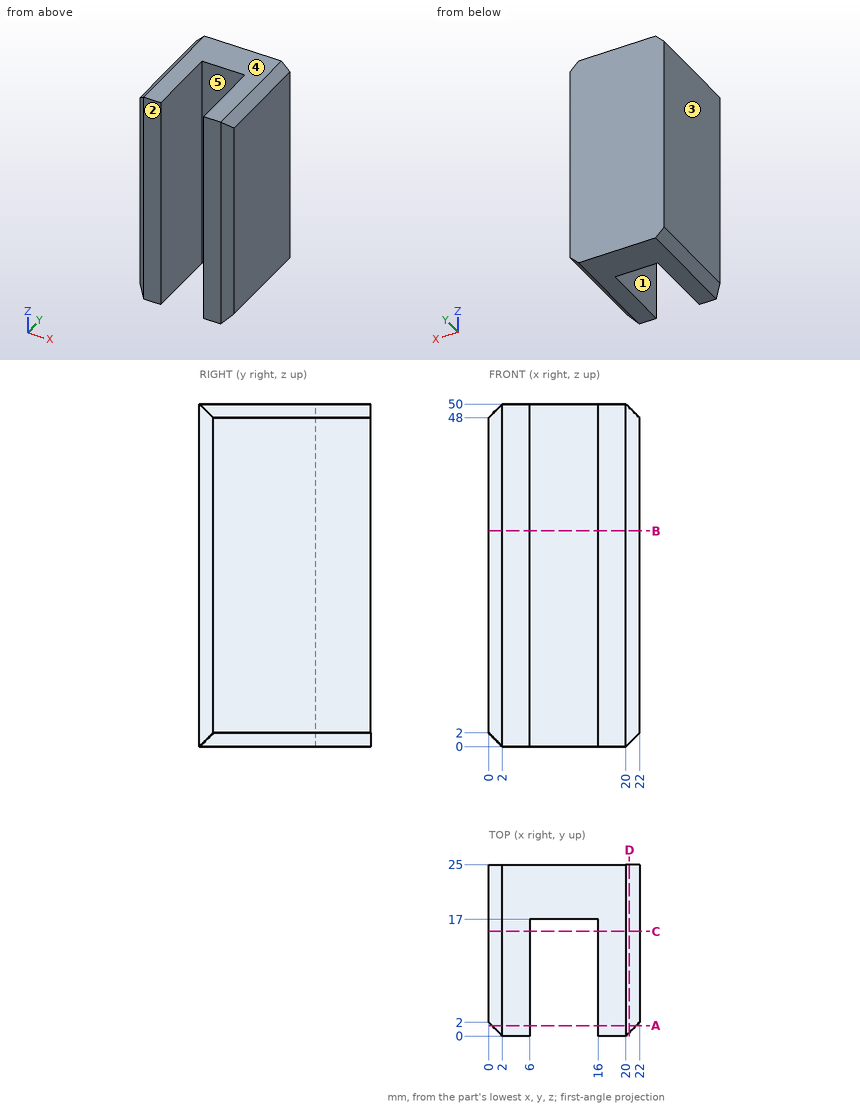
Can you work these out from the drawing? Everything is in mm from the part's minimum corner. A direction names the side the tool comes from. Round coordinates to 2 decimals unless told otherwise and drop trailing zeros. Loops run counter-clockwise (first coordinate to the right, second up) from the corner with the lowest first, then second, coordinate; pieces in that order, holes last.
1. If we section it at B-B on z = 31.5: Write out the boundary of the cut face in (x, y), plus the area to 3 significant figures.
Answer list:
outline: (0, 2) - (2, 0) - (6, 0) - (6, 17) - (16, 17) - (16, 0) - (20, 0) - (22, 2) - (22, 25) - (0, 25) - close
area: 376 mm2
2. If we section it at A-A on y = 1.5: Write out the boundary of the cut face in (x, z).
Answer list:
outline: (0.5, 1.5) - (2, 0) - (6, 0) - (6, 50) - (2, 50) - (0.5, 48.5) - close; (16, 0) - (20, 0) - (21.5, 1.5) - (21.5, 48.5) - (20, 50) - (16, 50) - close
3. We'd pull the mould along X, two halves only. Please class the marked faces 3, 4 and 5: +X half, -X half, draft (parallel to the pull), parting line (faces both ways), or undercut.
Answer list:
face 3: -X half
face 4: draft
face 5: undercut
4. If I drill on line 1 along X through (y, z) = (13.25, 12.5); line 2 along Y through (x, z) = (15.5, 12); line 3 along X through (y, z) = (1.75, 4), over which ranges is the centre line in solid material (lowest first)?
Answer list:
line 1: x = 0 to 6, 16 to 22
line 2: y = 17 to 25
line 3: x = 0.25 to 6, 16 to 21.75
5. For P1, Ø3, axis at x = 10.5, z = 16.5, coming from the -Y side, with a flat end and sliding along its axis, tell me the tip position at first contact or that it passes through.
Answer list:
P1: stops at y = 17
6. If we section it at D-D on x = 20.5: Write out the boundary of the cut face in (y, z).
Answer list:
outline: (0.5, 0.5) - (25, 0.5) - (25, 49.5) - (0.5, 49.5) - close
7. If we section it at C-C on y = 15.25: Write out the boundary of the cut face in (x, z).
Answer list:
outline: (0, 2) - (2, 0) - (6, 0) - (6, 50) - (2, 50) - (0, 48) - close; (16, 0) - (20, 0) - (22, 2) - (22, 48) - (20, 50) - (16, 50) - close
8. Which directions (+Z, -Z, +X, -X, +Y, -Y) give clear straight access to the entire face, cutting with the end or side of a thin tool? Please do the marked faces 1 and 2.
Answer list:
face 1: +Z, -Z, -Y
face 2: +Z, -Z, +X, -X, -Y
